For this review, use the dimensioned drawing (mm, ordinates from the lowest corner) and the shaded views. Round coordinates to 2 decimals unless told otherwise and drop trailing zeros. Loops run counter-clockwise (first coordinate to the right, second up) from the corner with the lowest first, then second, coordinate; pieces in that order, holes last. Notation, with made-up numbers: M 62.25,-39 L 117.25,-39 A32 cw 117.25,-7 Z; hole C 79.5,-25.75 d11. An arc over 180 degrees is marked long. Write item = value, one per line. Start each with the question number.
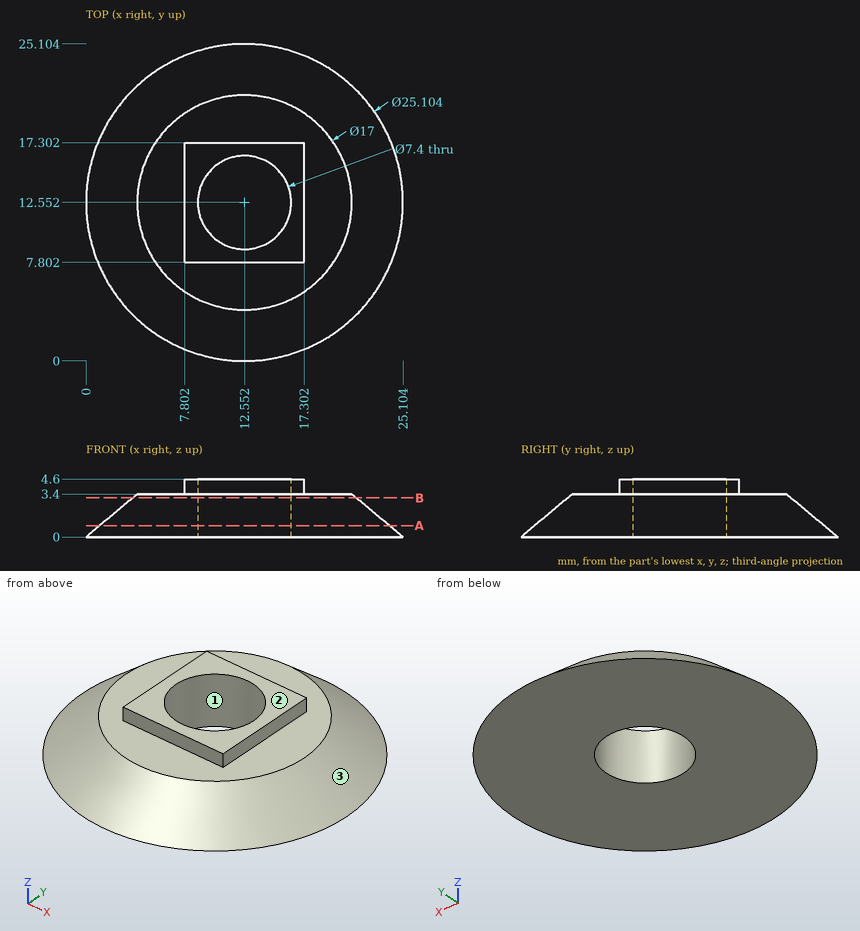
(1) Draft analysis for pull direction X (two halves, no side actions). For the marked faces 1, 2 and 3, state which applies: +X half, -X half, draft (parallel to the pull), parting line (faces both ways), or undercut.
(2) Wall thickness on L1, parallel to X at y = 14.5, z = 2.45 (1 decimal); L2, parallel to Z at x = 17.25, y = 6.75; L3, parallel to Y at x = 10.5, z = 2.25: over which ranges is each line inside the solid? List them lowest first.
(3) Add section B-B on z = 3.1. Write out the cut boundary in (x, y) (1 decimal), and give its area (3 significant figures).
(4) For pin 1 Ø0.6 at (x, z) = (15, 4) entering from -Y; pin 2 Ø1.3 at (y, z) = (11.5, 4) entering from +X; pin 3 Ø1.3 at (x, z) = (14.5, 4) entering from +Y, all flat-tipped, find the tip position at first contact; note any pin that passes through.
(5) Add section A-A on z = 0.9. Write out the cut boundary in (x, y), and give its area (3 significant figures).
Answer sheet:
q1.face_1 = undercut
q1.face_2 = draft
q1.face_3 = parting line
q2.L1 = 3.1 to 9.4, 15.7 to 22
q2.L2 = 0 to 3.4
q2.L3 = 2.9 to 9.47, 15.63 to 22.21
q3.outline = C 12.6,12.6 d17.7; hole C 12.6,12.6 d7.4
q3.area = 203 mm²
q4.pin_1 = 7.8
q4.pin_2 = 21.05
q4.pin_3 = 20.9
q5.outline = C 12.55,12.55 d22.96; hole C 12.55,12.55 d7.4
q5.area = 371 mm²
